Geometry: final body of the model. Coordinates: model frame, mm. A direction names the side the tool comes from. Coordinates: 2 decimals unless noted, no trailing zeros. Loops run counter-clockwise (first coordinate to the right, second up) from the corner with the lowest first, then second, coordinate; pieces in that order, holes last. Notation, with made-up numbers: (-13.75, 39.5) -> (-8.75, 39.5) arc R24 ccw to (-8.75, 52.5) -> close; hole circle Ø8 at (13.25, 38.25). An arc over 180 degrees is marked (long way). One line per item, written item: value. Start each with the question number.
from build123d import *

# Parameters (mm, degrees)
SKETCH1_W           = 9.1
SKETCH1_H           = 5.75
BOSS_EXTRUDE1_DEPTH = 2.2
SKETCH3_W           = 3.6
SKETCH3_H           = 5.75
BOSS_EXTRUDE2_DEPTH = 4
SKETCH2_W           = 1.60331862
SKETCH2_H           = 15
CUT_EXTRUDE1_DEPTH  = 3


with BuildPart() as part:
    # Sketch1 → Boss-Extrude1 (new body)
    with BuildSketch(Plane.XY):
        with Locations((-13.05, 11.375)):
            Rectangle(SKETCH1_W, SKETCH1_H)
    extrude(amount=BOSS_EXTRUDE1_DEPTH)

    # Sketch3 → Boss-Extrude2 (add)
    with BuildSketch(Plane(origin=(0, 0, 0), x_dir=(-1, 0, 0), z_dir=(0, 0, -1))):
        with Locations((13.05, 11.375)):
            Rectangle(SKETCH3_W, SKETCH3_H)
    extrude(amount=BOSS_EXTRUDE2_DEPTH)

    # Sketch2 → Cut-Extrude1 (cut)
    with BuildSketch(Plane.XY.offset(2.2)):
        with Locations((-13.05, 11.375)):
            Rectangle(SKETCH2_W, SKETCH2_H)
    extrude(amount=-CUT_EXTRUDE1_DEPTH, mode=Mode.SUBTRACT)


solid = part.part
1. Section B-B on y = 11.75. Return the cut outline in (x, z), plus the area to 3 significant figures.
2. Section D-D on z = -1.75. Return the cut outline in (x, y), plus the area to 3 significant figures.
3. Pin query (flat end, axial travel): pin 1 Ø0.8 at (x, y) = (-10, 10) entering from -Z; pin 2 Ø2 at (y, z) = (11.5, -2) entering from +X; pin 3 Ø0.8 at (x, y) = (-13, 10) entering from +Z. Return the tip coordinate at first contact, or that it passes through.
4. Draft query along X for faces 6 (the face through (-13.852, 11, 1)), 7 (the face through (-16, 11, 2.2)), 8 (the face through (-11.25, 11, -2)), 9 (the face through (-17.6, 11, 1)). Return one class per face: released by +X, released by -X, zero draft, split by the parting line, or undercut.
5. Line query: L1, parallel to X at y = 13.6, z = 1; L2, parallel to X at y = 9.25, z = -0.5; L3, parallel to X at y = 12.2, z = -2.25. Output: solid intervals per line, ascending. Write a range as [from, to].
6. Section A-A on z = 0.5. Return the cut outline in (x, y), plus the area to 3 significant figures.
7. Section C-C on z = -0.25. Return the cut outline in (x, y).
8. Set-up query: faces 1 (the face through (-16, 11, 0)), 2 (the face through (-8.5, 11, 1)), 3 (the face through (-13, 11, -0.8)), 4 (the face through (-13, 11, -4)), 5 (the face through (-10, 11, 0)). Return all of +Z, -Z, +X, -X, +Y, -Y with unobstructed straight access to the full face (end or side cutting, diameter ignored); none if empty.
Checks:
1. outline: (-17.6, 0) -> (-14.85, 0) -> (-14.85, -4) -> (-11.25, -4) -> (-11.25, 0) -> (-8.5, 0) -> (-8.5, 2.2) -> (-12.25, 2.2) -> (-12.25, -0.8) -> (-13.85, -0.8) -> (-13.85, 2.2) -> (-17.6, 2.2) -> close
1. area: 29.6 mm²
2. outline: (-14.85, 8.5) -> (-11.25, 8.5) -> (-11.25, 14.25) -> (-14.85, 14.25) -> close
2. area: 20.7 mm²
3. pin 1: z = 0
3. pin 2: x = -11.25
3. pin 3: z = -0.8
4. face 6: undercut
4. face 7: zero draft
4. face 8: released by +X
4. face 9: released by -X
5. L1: [-17.6, -13.85], [-12.25, -8.5]
5. L2: [-14.85, -13.85], [-12.25, -11.25]
5. L3: [-14.85, -11.25]
6. outline: (-17.6, 8.5) -> (-13.85, 8.5) -> (-13.85, 14.25) -> (-17.6, 14.25) -> close; (-12.25, 8.5) -> (-8.5, 8.5) -> (-8.5, 14.25) -> (-12.25, 14.25) -> close
6. area: 43.1 mm²
7. outline: (-14.85, 8.5) -> (-13.85, 8.5) -> (-13.85, 14.25) -> (-14.85, 14.25) -> close; (-12.25, 8.5) -> (-11.25, 8.5) -> (-11.25, 14.25) -> (-12.25, 14.25) -> close
8. face 1: -Z, -X, +Y, -Y
8. face 2: +Z, -Z, +X, +Y, -Y
8. face 3: +Z, +Y, -Y
8. face 4: -Z, +X, -X, +Y, -Y
8. face 5: -Z, +X, +Y, -Y
